Part model, mm, in its own coordinate system. A direction names the side the tool comes from. Coordinates: 2 decimals unless noted, no trailing zeros. Loops run counter-clockwise (first coordinate to the right, second up) from the corner with the lowest first, then second, coordinate; pieces in that order, holes last. Notation, with made-up numbers: (53.25, 63) - (79.25, 63) arc R28 ccw to (79.25, 101) - close; hole circle Ø2 at (-31.75, -28). An arc over 180 degrees is marked (long way). Use a Markdown table: item, result. Add a question column.
1. Band-saw the part on A-A, the plane z = 100. Give the cut face in (x, y).
2. 3-axis set-ups, long thin cutter, end or side, ignore diameter. For faces 4 (the flat face through (0, 0, 111.76)), 5 (the flat face through (0, 0, 0)): which of +Z, -Z, +X, -X, +Y, -Y reach the whole face in a straight line?
3. Drop flat-ended pins along their axis: pin 1 (2 mm diameter, centred on x = 16.5, z = 63.5, fed in from -Y); pin 2 (1.5 mm diameter, centred on x = -10, y = -9.5, fed in from +Z); pin 3 (6 mm diameter, centred on x = 19, z = 28.5, fed in from -Y); pin 4 (10 mm diameter, centred on x = 3.5, z = 90.5, fed in from -Y). Give the stop position or say it passes through.
4. Wall check: probe 1 along Z at (x, y) = (-4.5, -14); probe 2 along Y at (x, z) = (0, 113.3); probe 3 along Y at (x, z) = (0, 113). Give the ranges that are in metal, low to high. Write a range as [from, to].
5. Pull direction X, two halves, no side cores. Call faces 1 (the conical face through (22.11, 6.96, 113.98)), 2 (the cylindrical face through (11.63, 18.25, 113.05)), 3 (the flat face through (17, 14, 114.3)): pulls with the +X half, pulls with the -X half, needs draft (parallel to the pull), parting line crosses it, or undercut.
from build123d import *

# Parameters (mm, degrees)
F0_R     = 31.75
F1_DEPTH = 114.3
F2_SIZE  = 8.89
F3_SIZE  = 8.89
F4_R     = 7.62
F6_R     = 21.6402594839
F7_DEPTH = 2.54


with BuildPart() as f1:
    # F0 (on Top) → F1 (new body)
    with BuildSketch(Plane.XY):
        Circle(F0_R)
    extrude(amount=F1_DEPTH)

    # F2
    f2_edges = [f1.edges().sort_by_distance(p)[0] for p in [
        (-31.75, 0, 114.3),
    ]]
    chamfer(f2_edges, length=F2_SIZE)

    # F3
    f3_edges = [f1.edges().sort_by_distance(p)[0] for p in [
        (-31.75, 0, 0),
    ]]
    chamfer(f3_edges, length=F3_SIZE)

    # F4
    f4_edges = [f1.edges().sort_by_distance(p)[0] for p in [
        (-31.75, 0, 8.89),
        (-31.75, 0, 105.41),
    ]]
    fillet(f4_edges, radius=F4_R)

    # F6 (on face) → F7 (cut)
    with BuildSketch(Plane.XY.offset(114.3)):
        Circle(F6_R)
    extrude(amount=-F7_DEPTH, mode=Mode.SUBTRACT)


solid = f1.part
Geometry check:
| question | item | result |
|---|---|---|
| 1 | outline | circle Ø63.5 at (0, 0) |
| 2 | face 4 | +Z |
| 2 | face 5 | -Z, +X, -X, +Y, -Y |
| 3 | pin 1 | stops at y = -27.71 |
| 3 | pin 2 | stops at z = 111.76 |
| 3 | pin 3 | stops at y = -27.42 |
| 3 | pin 4 | stops at y = -31.75 |
| 4 | probe 1 | z = [0, 111.76] |
| 4 | probe 2 | y = [-23.86, -21.64], [21.64, 23.86] |
| 4 | probe 3 | y = [-24.16, -21.64], [21.64, 24.16] |
| 5 | face 1 | parting line crosses it |
| 5 | face 2 | undercut |
| 5 | face 3 | needs draft |
